from build123d import *

# Parameters (mm, degrees)
F0_W     = 40
F0_H     = 80
F1_DEPTH = 45
F3_D     = 8.8
F4_W     = 18
F4_H     = 52
F5_DEPTH = 45
F6_R     = 5


with BuildPart() as f1:
    # F0 (on Top) → F1 (new body)
    with BuildSketch(Plane.XY):
        with Locations((20, 40)):
            Rectangle(F0_W, F0_H)
    extrude(amount=F1_DEPTH)

    # F3 (through all)
    with Locations(Plane.XY.offset(45)):
        with Locations((30, 65), (30, 15)):
            Hole(F3_D / 2)

    # F4 (on face) → F5 (cut, through all)
    with BuildSketch(Plane.XY.offset(45)):
        with Locations((9, 40)):
            Rectangle(F4_W, F4_H)
    extrude(amount=-F5_DEPTH, mode=Mode.SUBTRACT)

    # F6
    f6_edges = [f1.edges().sort_by_distance(p)[0] for p in [
        (40, 0, 22.5),
        (40, 80, 22.5),
        (18, 14, 22.5),
        (18, 66, 22.5),
    ]]
    fillet(f6_edges, radius=F6_R)


solid = f1.part
Input: part model. Units: mm. Frame: model coordinates. A direction names the side the tool comes from. Give positions to 0.01 mm unless a question says otherwise; leave off trailing zeros. Order: outer loops, then holes, each group sorted by start corner. A loop starts at its lowest first (then second) coordinate and runs counter-clockwise, first axis right, second up.
Q1. Set-up query: faces 1 (the cylindrical face through (38, 1, 23)), 2 (the cylindrical face through (16, 15, 22)). Return all of +Z, -Z, +X, -X, +Y, -Y with unobstructed straight access to the full face (end or side cutting, diameter ignored); none if empty.
Checked values:
face 1: +Z, -Z, +X, -Y
face 2: +Z, -Z, -X
Q2. Ray query, probe 1 along Y at (x, z) = (30, 30); probe 2 along Y at (x, z) = (12, 38); probe 3 along Y at (x, z) = (28.5, 2.5). Return the intervals inside material, ascending.
Checked values:
probe 1: y = 0 to 10.6, 19.4 to 60.6, 69.4 to 80
probe 2: y = 0 to 14, 66 to 80
probe 3: y = 0 to 10.86, 19.14 to 60.86, 69.14 to 80
Q3. Draft query along X for faces 3 (the flat face through (18, 40, 23)), 4 (the flat face through (6, 66, 23)), 5 (the cylindrical face through (30.954, 60.705, 22.185)). Return one class per face: +X half, -X half, draft (parallel to the pull), parting line (faces both ways), or undercut.
Checked values:
face 3: -X half
face 4: draft
face 5: undercut
Q4. Contact query for a flat-ended pin moving along its axis: pin 1 Ø7 at (x, y) = (30, 65) entering from -Z. Output: stop coordinate, or through.
Checked values:
pin 1: passes through
Q5. Section C-C on x = 8.5. Output: boundary loops of the cut face in (y, z).
Checked values:
outline: (0, 0) - (14, 0) - (14, 45) - (0, 45) - close; (66, 0) - (80, 0) - (80, 45) - (66, 45) - close
Q6. Section B-B on y = 15. Output: boundary loops of the cut face in (x, z).
Checked values:
outline: (16, 0) - (25.6, 0) - (25.6, 45) - (16, 45) - close; (34.4, 0) - (40, 0) - (40, 45) - (34.4, 45) - close
Q7. Section D-D on z = 5. Output: boundary loops of the cut face in (x, y).
Checked values:
outline: (0, 0) - (35, 0) arc R5 ccw to (40, 5) - (40, 75) arc R5 ccw to (35, 80) - (0, 80) - (0, 66) - (13, 66) arc R5 cw to (18, 61) - (18, 19) arc R5 cw to (13, 14) - (0, 14) - close; hole circle Ø8.8 at (30, 15); hole circle Ø8.8 at (30, 65)
Q8. Section A-A on x = 30. Output: boundary loops of the cut face in (y, z).
Checked values:
outline: (0, 0) - (10.6, 0) - (10.6, 45) - (0, 45) - close; (19.4, 0) - (60.6, 0) - (60.6, 45) - (19.4, 45) - close; (69.4, 0) - (80, 0) - (80, 45) - (69.4, 45) - close
